from build123d import *

# Parameters (mm, degrees)
SKETCH3_R           = 63.246
SKETCH3_R_2         = 55.626
BOSS_EXTRUDE1_DEPTH = 63.5


# Read off the part's stored shape, not the designer's step: Shell1
with BuildPart() as part:
    # Sketch2 → Revolve1 (revolve)
    with BuildSketch(Plane.XY):
        with BuildLine():
            Line((-1295.2984, 0), (-1229.8934, 0))
            Line((-1229.8934, 0), (-1229.8934, 406.399027655))
            ThreePointArc((-1229.8934, 406.399027655), (-1278.842620934, 205.814226734), (-1295.2984, 0))
        make_face()
    revolve(axis=Axis((-1229.8934, 0, 0), (0, 1, 0)))

    # Shell1 outline → Shell1 (revolve, cut)
    with BuildSketch(Plane(origin=(-1229.8934, 0, 0), x_dir=(1, 0, 0), z_dir=(0, 0, 1))):
        with BuildLine():
            add(Edge.make_bspline(
                [(0, 381.415634791), (57.785, 195.085071394), (57.785, 0)],
                knots=[5.982469351, 5.982469351, 5.982469351, 6.283185307, 6.283185307, 6.283185307], degree=2, weights=[1, 0.988717519, 1]))
            Line((0, 381.415634791), (0, -1e-07))
            Line((0, -1e-07), (57.785, 0))
        make_face()
    revolve(axis=Axis((-1229.8934, 0, 0), (0, 1, 0)), mode=Mode.SUBTRACT)

    # Sketch3 → Boss-Extrude1 (add)
    with BuildSketch(Plane.XZ):
        with Locations(Location((-1229.8934, 0, 0), (0, 0, 270))):
            Circle(SKETCH3_R)
        with Locations(Location((-1229.8934, 0, 0), (0, 0, 270))):
            Circle(SKETCH3_R_2, mode=Mode.SUBTRACT)
    extrude(amount=BOSS_EXTRUDE1_DEPTH)


solid = part.part
Work out the finished part from the listing and answer in its coordinate system (mm). Coordinates: 2 decimals unless noted, no trailing zeros. One line per question, with ' | ' between items.
1) Consider probe 1 along X at (y, z) = (-29, 0); probe 2 along Z at (x, y) = (-1230.5, 95); probe 3 along Z at (x, y) = (-1184, 80). Determine where each line is inside the solid, lowest interval first. Write a range as [from, to].
Checks:
probe 1: [-1293.14, -1285.52], [-1174.27, -1166.65] | probe 2: [-61.91, -54.27], [54.27, 61.91] | probe 3: [-43.06, -30.85], [30.85, 43.06]
2) Flat-ended cylindrical pins translate along their axes: P1, Ø1.5, axis at x = -1268.5, y = 234.5, coming from the -Z side; P2, Ø12, axis at y = 254.5, z = 19, coming from the +X side; P3, Ø12, axis at x = -1276.5, y = 119.5, coming from the -Z side. Find the tip coordinate at first contact, or state that the pin passes through.
Checks:
P1: z = -22.46 | P2: x = -1191.55 | P3: z = -44.06
3) The mould has two halves that part along Z. Classify faces 1 (the face through (-1286, -63.5, 0)), 2 (the face through (-1291.635, -31.306, 13.71)), 3 (the face through (-1182.5, 0, 30.2)): +Z half, -Z half, draft (parallel to the pull), parting line (faces both ways), or undercut.
Checks:
face 1: draft | face 2: parting line | face 3: undercut
